Read the model definition and answer for the solid it produces. Units are mm, in the model's axes. A direction names the side the tool comes from. Give positions to 0.01 mm unless a question says otherwise; leave off trailing zeros. Order: outer loops, then holes, each group sorted by start corner. A loop starts at its lowest first (then second) coordinate and runs counter-clockwise, first axis right, second up. Notation, with made-up numbers: (0.25, -39.75) - (28.25, -39.75) arc R7 cw to (28.25, -29.75) - close; hole circle Ø9 at (-24.75, 58). An arc over 180 degrees is marked (long way). Write each question's results on one line, items separated by ' | '.
from build123d import *

# Parameters (mm, degrees)
BOSS_EXTRUDE1_DEPTH      = 9
BOSS_EXTRUDE1_DEPTH_BACK = 3
SKETCH1_W                = 4.9
SKETCH1_H                = 1.95
SKETCH2_W                = 4.9
SKETCH2_H                = 1.5
BOSS_EXTRUDE2_DEPTH      = 1.5
SKETCH3_W                = 10.45
SKETCH3_H                = 1.95
BOSS_EXTRUDE3_DEPTH      = 3.5
SKETCH4_W                = 7
SKETCH4_H                = 4.1
BOSS_EXTRUDE4_DEPTH      = 0.55


with BuildPart() as part:
    # Sketch1 → Boss-Extrude1 (new, two sides: drawn at the far end of the back side and taken through both)
    with BuildSketch(Plane.XY.offset(-BOSS_EXTRUDE1_DEPTH_BACK)):
        Rectangle(SKETCH1_W, SKETCH1_H)
    extrude(amount=BOSS_EXTRUDE1_DEPTH + BOSS_EXTRUDE1_DEPTH_BACK)

    # Sketch2 → Boss-Extrude2 (add)
    with BuildSketch(Plane(origin=(0, 0.975, 0), x_dir=(1, 0, 0), z_dir=(0, 1, 0))):
        with Locations((0, 2.25)):
            Rectangle(SKETCH2_W, SKETCH2_H)
    extrude(amount=BOSS_EXTRUDE2_DEPTH)

    # Sketch3 → Boss-Extrude3 (add, symmetric)
    with BuildSketch(Plane(origin=(0, 0, 0), x_dir=(0, 0, -1), z_dir=(1, 0, 0))):
        with Locations((-3.775, 0)):
            Rectangle(SKETCH3_W, SKETCH3_H)
    extrude(amount=BOSS_EXTRUDE3_DEPTH, both=True)

    # Sketch4 → Boss-Extrude4 (add)
    with BuildSketch(Plane(origin=(0, 0.975, 0), x_dir=(1, 0, 0), z_dir=(0, 1, 0))):
        with Locations((0, -6.95)):
            Rectangle(SKETCH4_W, SKETCH4_H)
    extrude(amount=BOSS_EXTRUDE4_DEPTH)


solid = part.part
(1) Section C-C (z = -0.75) is taken. Give the vertices of the cut face in (x, y) (3 decimals).
Conclusion:
outline: (-3.5, -0.975) - (3.5, -0.975) - (3.5, 0.975) - (-3.5, 0.975) - close
(2) Each of these flat-tipped pins is pushed along its axis until it touches: pin 1 (1.2 mm diameter, centred on x = 1, z = 6.5, fed in from +Y) (3 decimals); pin 2 (0.5 mm diameter, centred on y = 0.5, z = -2, fed in from +X); pin 3 (3 mm diameter, centred on x = -0.5, z = 1, fed in from +Y) (3 decimals). Where does it stop, or does it pass through?
Conclusion:
pin 1: y = 1.525 | pin 2: x = 2.45 | pin 3: y = 0.975
(3) Section B-B (x = 1.25) is taken. Give the vertices of the cut face in (y, z) (3 decimals), plus the area to 3 significant figures.
Conclusion:
outline: (-0.975, -3) - (2.475, -3) - (2.475, -1.5) - (0.975, -1.5) - (0.975, 4.9) - (1.525, 4.9) - (1.525, 9) - (-0.975, 9) - close | area: 27.9 mm^2
(4) Section A-A (y = 1.1) is taken. Give the vertices of the cut face in (x, z), plus the area to 4 significant figures.
Conclusion:
outline: (-3.5, 4.9) - (3.5, 4.9) - (3.5, 9) - (-3.5, 9) - close; (-2.45, -3) - (2.45, -3) - (2.45, -1.5) - (-2.45, -1.5) - close | area: 36.05 mm^2
(5) For faces 1 (the face through (0, 2, -1.5)), 2 (the face through (-3, 0, -1.45)), 3 (the face through (0, 1.525, 7)), 4 (the face through (0, 1, -3)), 5 (the face through (2.45, 1, -2)), determine the directions among +Z, -Z, +X, -X, +Y, -Y from which every point of the face is accessible in a straight line to the end or side of a thin tool.
Conclusion:
face 1: +X, -X, +Y | face 2: -Z, -X, +Y, -Y | face 3: +Z, +X, -X, +Y | face 4: -Z, +X, -X, +Y, -Y | face 5: -Z, +X, +Y, -Y
(6) Section D-D (z = 6.75) is taken. Give the vertices of the cut face in (x, y) (3 decimals), plus the area to 3 significant figures.
Conclusion:
outline: (-3.5, -0.975) - (3.5, -0.975) - (3.5, 1.525) - (-3.5, 1.525) - close | area: 17.5 mm^2
(7) Consider probe 1 along Z at (x, y) = (1.75, 1.1); probe 2 along Y at (x, z) = (0.75, 7.5) (3 decimals); probe 3 along Y at (x, z) = (-2.25, 4.5) (3 decimals). Determine where each line is inside the solid, lowest interval first. Write a range as [from, to].
Conclusion:
probe 1: [-3, -1.5], [4.9, 9] | probe 2: [-0.975, 1.525] | probe 3: [-0.975, 0.975]
(8) The mould has two halves that part along Z. Classify faces 6 (the face through (0, 0, 9)), 7 (the face through (0, 0.975, 2)), 8 (the face through (0, 2.475, -2)): pulls with the +Z half, pulls with the -Z half, needs draft (parallel to the pull), parting line crosses it, or undercut.
Conclusion:
face 6: pulls with the +Z half | face 7: undercut | face 8: needs draft
